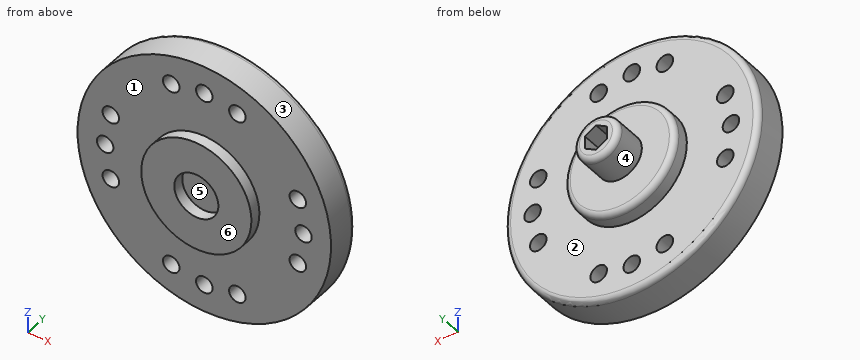
from build123d import *

# Parameters (mm, degrees)
CROQUIS1_R              = 11.5
SALIENTE_EXTRUIR1_DEPTH = 3
CROQUIS1_9_R            = 0.75
CORTAR_EXTRUIR2_DEPTH   = 3
MATRIZC2_COUNT          = 4
SALIENTE_EXTRUIR2_START = 3
CROQUIS1_11_R           = 5
SALIENTE_EXTRUIR2_DEPTH = 1.5
SALIENTE_EXTRUIR3_START = 4.5
CROQUIS1_12_R           = 2
SALIENTE_EXTRUIR3_DEPTH = 3
REDONDEO1_R             = 0.5
SALIENTE_EXTRUIR4_START = -1
CROQUIS1_13_R           = 5
CROQUIS1_13_R_2         = 2
SALIENTE_EXTRUIR4_DEPTH = 1


with BuildPart() as part:
    # Croquis1 → Saliente-Extruir1 (new body)
    with BuildSketch(Plane(origin=(0, 0, 0), x_dir=(1, 0, 0), z_dir=(0, 1, 0))):
        with Locations(Location((0, 13.3, 0), (0, 0, 270))):
            Circle(CROQUIS1_R)
    extrude(amount=SALIENTE_EXTRUIR1_DEPTH)

    # Croquis1<9> → Cortar-Extruir2 (cut)
    with BuildSketch(Plane(origin=(0, 0, 0), x_dir=(1, 0, 0), z_dir=(0, 1, 0))):
        with Locations(Location((0, 22.3, 0), (0, 0, 270))):
            Circle(CROQUIS1_9_R)
        with Locations(Location((3, 21.785281374, 0), (0, 0, 270))):
            Circle(CROQUIS1_9_R)
        with Locations(Location((-3, 21.785281374, 0), (0, 0, 90))):
            Circle(CROQUIS1_9_R)
    cortar_extruir2 = extrude(amount=CORTAR_EXTRUIR2_DEPTH, mode=Mode.SUBTRACT)

    # MatrizC2: Cortar-Extruir2 ×4 about axis
    matrizc2_axis = Axis((0, 0, -13.3), (0, 1, 0))
    for i in range(1, MATRIZC2_COUNT):
        add(cortar_extruir2.rotate(matrizc2_axis, i * 360 / MATRIZC2_COUNT), mode=Mode.SUBTRACT)

    # Croquis1<11> → Saliente-Extruir2 (add)
    with BuildSketch(Plane(origin=(0, 0, 0), x_dir=(1, 0, 0), z_dir=(0, 1, 0)).offset(SALIENTE_EXTRUIR2_START)):
        with Locations(Location((0, 13.3, 0), (0, 0, 270))):
            Circle(CROQUIS1_11_R)
    extrude(amount=SALIENTE_EXTRUIR2_DEPTH)

    # Croquis1<12> → Saliente-Extruir3 (add)
    with BuildSketch(Plane(origin=(0, 0, 0), x_dir=(1, 0, 0), z_dir=(0, 1, 0)).offset(SALIENTE_EXTRUIR3_START)):
        with Locations(Location((0, 13.3, 0), (0, 0, 270))):
            Circle(CROQUIS1_12_R)
        Polygon((1, 12.722649731), (1, 13.877350269), (0, 14.454700538), (-1, 13.877350269), (-1, 12.722649731), (0, 12.145299462), align=None, mode=Mode.SUBTRACT)
    extrude(amount=SALIENTE_EXTRUIR3_DEPTH)

    # Redondeo1
    redondeo1_edges = [part.edges().sort_by_distance(p)[0] for p in [
        (0, 3, -24.8),
        (0, 4.5, -18.3),
        (0, 7.5, -15.3),
    ]]
    fillet(redondeo1_edges, radius=REDONDEO1_R)

    # Croquis1<13> → Saliente-Extruir4 (add)
    with BuildSketch(Plane(origin=(0, 0, 0), x_dir=(1, 0, 0), z_dir=(0, 1, 0)).offset(SALIENTE_EXTRUIR4_START)):
        with Locations(Location((0, 13.3, 0), (0, 0, 270))):
            Circle(CROQUIS1_13_R)
        with Locations(Location((0, 13.3, 0), (0, 0, 270))):
            Circle(CROQUIS1_13_R_2, mode=Mode.SUBTRACT)
    extrude(amount=SALIENTE_EXTRUIR4_DEPTH)


solid = part.part
Check sheet for the modelled part. Datum: model origin and axes. Units: mm. Face numbers are marked on the shaded views. A direction names the side the tool comes from. Coordinates: 2 decimals unless noted, no trailing zeros. Write each loop counter-clockwise with the first axis right and the second up, starting at its lowest first coordinate (ties: lowest second). Pieces come first, ordered by that corner, then holes.
Item 1: Access from +Z, -Z, +X, -X, +Y, -Y to the whole of each face (thin tool, end or side, straight path). Record for the marked faces 1, 2 and 3.
Numbers:
face 1: -Y
face 2: +Y
face 3: +Y, -Y
Item 2: Cross-section at A-A on z = -13.3. Count the separate pieces of the cut face and the enclosed holes in it, then the cut area to 3 significant figures.
Numbers:
separate pieces: 3
enclosed holes: 0
area: 86.7 mm2
Item 3: Scan lines: probe 1 along X at (y, z) = (1.45, -16.3); probe 2 along Z at (x, y) = (-0.5, 0.5); probe 3 along X at (y, z) = (1, -4.3). Record each from-to range of solid material in increasing order.
Numbers:
probe 1: x = -11.1 to -9.24, -7.74 to 7.74, 9.24 to 11.1
probe 2: z = -24.79 to -22.86, -21.74 to -4.86, -3.74 to -1.81
probe 3: x = -7.16 to -3.55, -2.45 to -0.75, 0.75 to 2.45, 3.55 to 7.16
Item 4: Depth check by flat-ended pin: pin 1 Ø2 at (x, z) = (-8.49, -10.3) entering from -Y; pin 2 Ø1.4 at (x, z) = (-9, -13.3) entering from -Y; pin 3 Ø5 at (y, z) = (0.5, -18.5) entering from -X; pin 4 Ø3 at (y, z) = (1, -17) entering from -X. Enter the tip coordinate at first touch or a pass-through.
Numbers:
pin 1: stops at y = 0
pin 2: passes through
pin 3: stops at x = -11.18
pin 4: stops at x = -11.29
Item 5: Cross-section at B-B on y = 3.5. Record the boundary of the cut face in (x, z).
Numbers:
outline: circle Ø10 at (0, -13.3)
Item 6: Mould release check, pull along X, two halves, no side actions. Record for the marked faces 4, 5 and 6: released by +X, released by -X, zero draft, split by the parting line, or undercut.
Numbers:
face 4: split by the parting line
face 5: undercut
face 6: zero draft
